Read the model definition and answer for the solid it produces. Units are mm, in the model's axes. A direction names the side the tool comes from. Round coordinates to 2 decimals unless told otherwise and drop trailing zeros. Write each loop counter-clockwise with the first axis right and the second up, starting at its lowest first coordinate (ties: lowest second). Pieces come first, ordered by that corner, then holes. Notation, with made-up numbers: (-1, 64.5) -> (48, 64.5) arc R20 cw to (48, 82.5) -> close; hole circle Ø8 at (49, 28.5). An arc over 180 degrees is marked (long way). Return JSON: item names as keys, results as strings.
from build123d import *

# Parameters (mm, degrees)
SKETCH2_W             = 10
SKETCH2_H             = 14
SKETCH2_R             = 2.1
BOSS_EXTRUDE1_DEPTH   = 5
BOSS_EXTRUDE1_2_DEPTH = 5
SKETCH3_W             = 44.5
SKETCH3_H             = 39
SKETCH3_W_2           = 14
SKETCH3_H_2           = 5
BOSS_EXTRUDE2_DEPTH   = 2
BOSS_EXTRUDE4_DEPTH   = 32
SKETCH5_W             = 2
SKETCH5_H             = 85
BOSS_EXTRUDE5_DEPTH   = 37
SKETCH6_W             = 14
SKETCH6_H             = 30
CUT_EXTRUDE1_DEPTH    = 200
SKETCH7_W             = 20
SKETCH7_H             = 20
CUT_EXTRUDE2_DEPTH    = 16
FILLET1_R             = 2
SKETCH8_W             = 119.619460544
SKETCH8_H             = 55.607641494
CUT_EXTRUDE3_DEPTH    = 32
SKETCH9_W             = 100
SKETCH9_H             = 35
BOSS_EXTRUDE6_DEPTH   = 2
SKETCH10_W            = 89
SKETCH10_H            = 4
CUT_EXTRUDE4_DEPTH    = 10
BOSS_EXTRUDE7_DEPTH   = 25
SKETCH12_W            = 2
SKETCH12_H            = 35
BOSS_EXTRUDE8_DEPTH   = 2
SKETCH13_W            = 104
SKETCH13_H            = 37
BOSS_EXTRUDE9_DEPTH   = 2
SKETCH14_W            = 13
SKETCH14_H            = 30
CUT_EXTRUDE5_DEPTH    = 104
SKETCH15_W            = 113.891819436
SKETCH15_H            = 51.603678666
CUT_EXTRUDE6_DEPTH    = 27
SKETCH16_W            = 114.232812907
SKETCH16_H            = 49.785046819
CUT_EXTRUDE7_DEPTH    = 2
SKETCH17_W            = 89
SKETCH17_H            = 39
BOSS_EXTRUDE10_DEPTH  = 34
SKETCH18_W            = 30
SKETCH18_H            = 85
CUT_EXTRUDE8_DEPTH    = 37
SKETCH19_W            = 7
SKETCH19_H            = 30
CUT_EXTRUDE9_DEPTH    = 93
CUT_EXTRUDE10_DEPTH   = 17


with BuildPart() as part:
    # Sketch2 → Boss-Extrude1 (new body)
    with BuildSketch(Plane(origin=(0, 0, 0), x_dir=(1, 0, 0), z_dir=(0, 1, 0))):
        with Locations((114.448385229, -132.360414745)):
            Rectangle(SKETCH2_W, SKETCH2_H)
        with Locations((114.448385229, -132.360414745)):
            Circle(SKETCH2_R, mode=Mode.SUBTRACT)
    extrude(amount=BOSS_EXTRUDE1_DEPTH)



with BuildPart() as body_2:
    # Sketch2 → Boss-Extrude1 2 (new body)
    with BuildSketch(Plane(origin=(0, 0, 0), x_dir=(1, 0, 0), z_dir=(0, 1, 0))):
        with Locations((114.448385229, -172.360414745)):
            Rectangle(SKETCH2_W, SKETCH2_H)
        with Locations((114.448385229, -172.360414745)):
            Circle(SKETCH2_R, mode=Mode.SUBTRACT)
    extrude(amount=BOSS_EXTRUDE1_2_DEPTH)


with BuildPart() as part_1:
    add(part.part)

    add(body_2.part)  # Boss-Extrude2 merges body 2
    # Sketch3 → Boss-Extrude2 (add)
    with BuildSketch(Plane(origin=(119.448385229, 0, 0), x_dir=(0, 0, -1), z_dir=(1, 0, 0))):
        Polygon((-152.360414745, -34), (-152.360414745, 5), (-165.360414745, 5), (-165.360414745, 0), (-179.360414745, 0), (-179.360414745, 5), (-196.860414745, 5), (-196.860414745, -34), align=None)
        with Locations((-130.110414745, -14.5)):
            Rectangle(SKETCH3_W, SKETCH3_H)
        with Locations((-172.360414745, 2.5)):
            Rectangle(SKETCH3_W_2, SKETCH3_H_2)
    extrude(amount=BOSS_EXTRUDE2_DEPTH)

    # Sketch4 → Boss-Extrude4 (add)
    with BuildSketch(Plane(origin=(121.448385229, 0, 0), x_dir=(0, 0, -1), z_dir=(1, 0, 0))):
        Polygon((-194.860414745, 5), (-196.860414745, 5), (-196.860414745, -34), (-107.860414745, -34), (-107.860414745, 5), (-109.860414745, 5), (-109.860414745, -32), (-194.860414745, -32), align=None)
    extrude(amount=BOSS_EXTRUDE4_DEPTH)

    # Sketch5 → Boss-Extrude5 (add)
    with BuildSketch(Plane(origin=(0, -32, 0), x_dir=(1, 0, 0), z_dir=(0, 1, 0))):
        with Locations((152.448385229, -152.360414745)):
            Rectangle(SKETCH5_W, SKETCH5_H)
    extrude(amount=BOSS_EXTRUDE5_DEPTH)

    # Sketch6 → Cut-Extrude1 (cut)
    with BuildSketch(Plane.XY.offset(196.860414745)):
        with Locations((136.448385229, -10)):
            Rectangle(SKETCH6_W, SKETCH6_H)
    extrude(amount=-CUT_EXTRUDE1_DEPTH, mode=Mode.SUBTRACT)

    # Sketch7 → Cut-Extrude2 (cut)
    with BuildSketch(Plane(origin=(153.448385229, 0, 0), x_dir=(0, 0, -1), z_dir=(1, 0, 0))):
        with Locations((-179.360414745, -14.5)):
            Rectangle(SKETCH7_W, SKETCH7_H)
        with Locations((-152.360414745, -14.5)):
            Rectangle(SKETCH7_W, SKETCH7_H)
        with Locations((-125.360414745, -14.5)):
            Rectangle(SKETCH7_W, SKETCH7_H)
    extrude(amount=-CUT_EXTRUDE2_DEPTH, mode=Mode.SUBTRACT)

    # Fillet1
    fillet1_edges = [part_1.edges().sort_by_distance(p)[0] for p in [
        (109.448385229, 2.5, 139.360414745),
        (109.448385229, 2.5, 125.360414745),
        (109.448385229, 2.5, 179.360414745),
        (109.448385229, 2.5, 165.360414745),
    ]]
    fillet(fillet1_edges, radius=FILLET1_R)

    # Sketch8 → Cut-Extrude3 (cut)
    with BuildSketch(Plane(origin=(153.448385229, 0, 0), x_dir=(0, 0, -1), z_dir=(1, 0, 0))):
        with Locations((-148.578534845, -15.335015755)):
            Rectangle(SKETCH8_W, SKETCH8_H)
    extrude(amount=-CUT_EXTRUDE3_DEPTH, mode=Mode.SUBTRACT)

    # Sketch9 → Boss-Extrude6 (add)
    with BuildSketch(Plane(origin=(121.448385229, 0, 0), x_dir=(0, 0, -1), z_dir=(1, 0, 0))):
        with Locations((-152.360414745, -12.5)):
            Rectangle(SKETCH9_W, SKETCH9_H)
    extrude(amount=-BOSS_EXTRUDE6_DEPTH)

    # Sketch10 → Cut-Extrude4 (cut)
    with BuildSketch(Plane(origin=(121.448385229, 0, 0), x_dir=(0, 0, -1), z_dir=(1, 0, 0))):
        with Locations((-152.360414745, -32)):
            Rectangle(SKETCH10_W, SKETCH10_H)
    extrude(amount=-CUT_EXTRUDE4_DEPTH, mode=Mode.SUBTRACT)



with BuildPart() as body_2_2:
    # Sketch11 → Boss-Extrude7 (new body)
    with BuildSketch(Plane(origin=(121.448385229, 0, 0), x_dir=(0, 0, -1), z_dir=(1, 0, 0))):
        Polygon((-202.360414745, -30), (-202.360414745, 5), (-204.360414745, 5), (-204.360414745, -32), (-100.360414745, -32), (-100.360414745, 5), (-102.360414745, 5), (-102.360414745, -30), align=None)
    extrude(amount=BOSS_EXTRUDE7_DEPTH)


with BuildPart() as part_2:
    add(part_1.part)

    add(body_2_2.part)  # Boss-Extrude8 merges body 2 2
    # Sketch12 → Boss-Extrude8 (add)
    with BuildSketch(Plane.ZY.offset(-121.448385229)):
        with Locations((101.360414745, -12.5)):
            Rectangle(SKETCH12_W, SKETCH12_H)
        Polygon((102.360414745, -30), (100.360414745, -30), (100.360414745, -32), (204.360414745, -32), (204.360414745, -30), (202.360414745, -30), align=None)
        with Locations((203.360414745, -12.5)):
            Rectangle(SKETCH12_W, SKETCH12_H)
    extrude(amount=BOSS_EXTRUDE8_DEPTH)

    # Sketch13 → Boss-Extrude9 (add)
    with BuildSketch(Plane(origin=(146.448385229, 0, 0), x_dir=(0, 0, -1), z_dir=(1, 0, 0))):
        with Locations((-152.360414745, -13.5)):
            Rectangle(SKETCH13_W, SKETCH13_H)
        Polygon((-195.798080738, -22), (-175.798080738, -22), (-185.798080738, -0.554930795), align=None, mode=Mode.SUBTRACT)
        Polygon((-128.922748753, -22), (-118.922748753, -0.554930795), (-108.922748753, -22), align=None, mode=Mode.SUBTRACT)
        Polygon((-162.360414745, -22), (-142.360414745, -22), (-152.360414745, -0.554930795), align=None, mode=Mode.SUBTRACT)
    extrude(amount=BOSS_EXTRUDE9_DEPTH)

    # Sketch14 → Cut-Extrude5 (cut)
    with BuildSketch(Plane(origin=(0, 0, 100.360414745), x_dir=(-1, 0, 0), z_dir=(0, 0, -1))):
        with Locations((-133.948385229, 5)):
            Rectangle(SKETCH14_W, SKETCH14_H)
    extrude(amount=-CUT_EXTRUDE5_DEPTH, mode=Mode.SUBTRACT)

    # Sketch15 → Cut-Extrude6 (cut)
    with BuildSketch(Plane(origin=(148.448385229, 0, 0), x_dir=(0, 0, -1), z_dir=(1, 0, 0))):
        with Locations((-152.246750255, -13.320211528)):
            Rectangle(SKETCH15_W, SKETCH15_H)
    extrude(amount=-CUT_EXTRUDE6_DEPTH, mode=Mode.SUBTRACT)

    # Sketch16 → Cut-Extrude7 (cut)
    with BuildSketch(Plane(origin=(121.448385229, 0, 0), x_dir=(0, 0, -1), z_dir=(1, 0, 0))):
        with Locations((-151.848924539, -14.329503265)):
            Rectangle(SKETCH16_W, SKETCH16_H)
    extrude(amount=-CUT_EXTRUDE7_DEPTH, mode=Mode.SUBTRACT)

    # Sketch17 → Boss-Extrude10 (add)
    with BuildSketch(Plane(origin=(119.448385229, 0, 0), x_dir=(0, 0, -1), z_dir=(1, 0, 0))):
        with Locations((-152.360414745, -14.5)):
            Rectangle(SKETCH17_W, SKETCH17_H)
    extrude(amount=BOSS_EXTRUDE10_DEPTH)

    # Sketch18 → Cut-Extrude8 (cut)
    with BuildSketch(Plane(origin=(0, 5, 0), x_dir=(1, 0, 0), z_dir=(0, 1, 0))):
        with Locations((136.448385229, -152.360414745)):
            Rectangle(SKETCH18_W, SKETCH18_H)
    extrude(amount=-CUT_EXTRUDE8_DEPTH, mode=Mode.SUBTRACT)

    # Sketch19 → Cut-Extrude9 (cut)
    with BuildSketch(Plane.XY.offset(196.860414745)):
        with Locations((132.948385229, -10)):
            Rectangle(SKETCH19_W, SKETCH19_H)
        with Locations((139.948385229, -10)):
            Rectangle(SKETCH19_W, SKETCH19_H)
    extrude(amount=-CUT_EXTRUDE9_DEPTH, mode=Mode.SUBTRACT)

    # Sketch20 → Cut-Extrude10 (cut)
    with BuildSketch(Plane(origin=(153.448385229, 0, 0), x_dir=(0, 0, -1), z_dir=(1, 0, 0))):
        Polygon((-186.860414745, -25.637480673), (-161.860414745, -25.637480673), (-174.360414745, -0.637480673), align=None)
        Polygon((-117.860414745, -25.637480673), (-142.860414745, -25.637480673), (-130.360414745, -0.637480673), align=None)
    extrude(amount=-CUT_EXTRUDE10_DEPTH, mode=Mode.SUBTRACT)


solid = part_2.part
Item 1: Section B-B (y = -22.5) is taken. Give the vertices of the cut face in (x, z).
Worked answers:
{"outline": "(119.45, 107.86) -> (129.45, 107.86) -> (129.45, 109.86) -> (121.45, 109.86) -> (121.45, 194.86) -> (129.45, 194.86) -> (129.45, 196.86) -> (119.45, 196.86) -> close; (143.45, 107.86) -> (153.45, 107.86) -> (153.45, 119.43) -> (151.45, 119.43) -> (151.45, 109.86) -> (143.45, 109.86) -> close; (143.45, 194.86) -> (151.45, 194.86) -> (151.45, 185.29) -> (153.45, 185.29) -> (153.45, 196.86) -> (143.45, 196.86) -> close; (151.45, 141.29) -> (153.45, 141.29) -> (153.45, 163.43) -> (151.45, 163.43) -> close"}
Item 2: Section A-A (x = 117.5) is taken. Give the vertices of the cut face in (y, z), then the cut area to 3 significant figures.
Worked answers:
{"outline": "(0, 125.36) -> (5, 125.36) -> (5, 139.36) -> (0, 139.36) -> close; (0, 165.36) -> (5, 165.36) -> (5, 179.36) -> (0, 179.36) -> close", "area": "140 mm2"}
Item 3: A tool of negligible diameter and unlimited length cuts with its end or side. For faces 4 (the cylindrical face through (110.05, 2.54, 138.79)), 5 (the flat face through (136, -25, 196)), 6 (the flat face through (117, 0, 132)), from which of +Z, -Z, +X, -X, +Y, -Y can it reach the whole face along a straight path? Write none if from no direction.
Worked answers:
{"face 4": "-X, +Y, -Y", "face 5": "+Z, -Z, +Y", "face 6": "+Z, -Z, -X, -Y"}
Item 4: Flat-ended cylindrical pins translate along their axes: pin 1 (4 mm diameter, centred on x = 114.45, z = 132.36, fed in from -Y); pin 2 (2 mm diameter, centred on x = 149, z = 181.5, fed in from +Y); pin 3 (8 mm diameter, centred on x = 114.5, z = 132.5, fed in from -Y); pin 4 (5.5 mm diameter, centred on x = 116.5, y = 2.5, fed in from -Z). Find the tip coordinate at first contact, or state that the pin passes through.
Worked answers:
{"pin 1": "passes through", "pin 2": "stops at y = -32", "pin 3": "stops at y = 0", "pin 4": "stops at z = 125.36"}
Item 5: Section C-C (z = 151) is taken. Give the vertices of the cut face in (x, y).
Worked answers:
{"outline": "(119.45, -34) -> (153.45, -34) -> (153.45, 5) -> (151.45, 5) -> (151.45, -32) -> (121.45, -32) -> (121.45, 5) -> (119.45, 5) -> close"}
Item 6: Section D-D (x = 146) is taken. Give the vertices of the cut face in (y, z), then the cut area to 3 significant figures.
Worked answers:
{"outline": "(-34, 107.86) -> (5, 107.86) -> (5, 109.86) -> (-32, 109.86) -> (-32, 194.86) -> (5, 194.86) -> (5, 196.86) -> (-34, 196.86) -> close", "area": "326 mm2"}
Item 7: For a pull along X with two mould halves and no side action, classify faces 1 (the flat face through (152.462, -13.312, 136.698)), 2 (the cylindrical face through (110.05, 2.54, 178.79)), 3 (the flat face through (121.448, -13, 153)) as released by +X, released by -X, zero draft, split by the parting line, or undercut.
Worked answers:
{"face 1": "zero draft", "face 2": "released by -X", "face 3": "undercut"}
Item 8: Straight lines are drawn through the part: L1, parallel to Z at x = 123.5, y = -13.5; L2, parallel to X at y = -29, z = 193; L3, parallel to X at y = -21, z = 182. For each, find the intervals that lie inside material, in ascending order. Write a range as [from, to].
Worked answers:
{"L1": "z = [107.86, 109.86], [194.86, 196.86]", "L2": "x = [119.45, 121.45], [151.45, 153.45]", "L3": "x = [119.45, 121.45]"}
